from build123d import *

# Parameters (mm, degrees)
SKETCH_1_W           = 20
SKETCH_1_H           = 15
EXTRUDE_1_DEPTH      = 30
EXTRUDE_2_DEPTH      = 6
EXTRUDE_2_DEPTH_BACK = 6
SKETCH_3_R           = 1.35
EXTRUDE_3_DEPTH      = 11.5
EXTRUDE_START        = -0.2
EXTRUDE_4_DEPTH      = 29.6
EXTRUDE_5_DEPTH      = 14.6
FILLET_1_R           = 0.1
FILLET_2_R           = 0.2
SKETCH_6_R           = 1.25
CUT_EXTRUDE_1_DEPTH  = 38.165171868
SKETCH_7_R           = 1.25
CUT_EXTRUDE_2_DEPTH  = 40.449334595
SKETCH_8_R           = 1.25
CUT_EXTRUDE_3_DEPTH  = 5


with BuildPart() as part:
    # 草图1 → 凸台-拉伸1 (new body)
    with BuildSketch(Plane.XY):
        Rectangle(SKETCH_1_W, SKETCH_1_H)
    extrude(amount=-EXTRUDE_1_DEPTH)

    # 草图2 → 凸台-拉伸2 (add, two sides: drawn at the far end of the back side and taken through both)
    with BuildSketch(Plane(origin=(0, 0, 0), x_dir=(1, 0, 0), z_dir=(0, 1, 0)).offset(-EXTRUDE_2_DEPTH_BACK)):
        with BuildLine():
            Line((-4.25, 0), (-5.75, 0))
            Line((-5.75, 0), (-5.75, -0.638562172))
            ThreePointArc((-5.75, -0.638562172), (-5, -2.3), (-4.25, -0.638562172))
            Line((-4.25, -0.638562172), (-4.25, 0))
        make_face()
        with BuildLine():
            Line((4.25, 0), (4.25, -0.638562172))
            ThreePointArc((4.25, -0.638562172), (5, -2.3), (5.75, -0.638562172))
            Line((5.75, -0.638562172), (5.75, 0))
            Line((5.75, 0), (4.25, 0))
        make_face()
    extrude(amount=EXTRUDE_2_DEPTH + EXTRUDE_2_DEPTH_BACK)

    # 草图3 → 凸台-拉伸3 (add)
    with BuildSketch(Plane.XY):
        with Locations(Location((0, 0, 0), (0, 0, 180))):
            Circle(SKETCH_3_R)
    extrude(amount=EXTRUDE_3_DEPTH)

    # 草图4 → 凸台-拉伸4 (add)
    with BuildSketch(Plane.XY.offset(EXTRUDE_START)):
        with BuildLine():
            Line((-1.5, 7.5), (-1.5, 8.177124344))
            ThreePointArc((-1.5, 8.177124344), (-1.780042303, 8.588161527), (-1.95, 9.055590279))
            Line((-1.95, 9.055590279), (-1.95, 10))
            Line((-1.95, 10), (-1.165769145, 10))
            Line((-1.165769145, 10), (-0.5, 8.57225346))
            Line((-0.5, 8.57225346), (-0.5, 7.5))
            Line((-0.5, 7.5), (-1.5, 7.5))
        make_face()
        with BuildLine():
            Line((1.5, 7.5), (1.5, 8.177124344))
            ThreePointArc((1.5, 8.177124344), (1.780042303, 8.588161527), (1.95, 9.055590279))
            Line((1.95, 9.055590279), (1.95, 10))
            Line((1.95, 10), (1.165769145, 10))
            Line((1.165769145, 10), (0.5, 8.57225346))
            Line((0.5, 8.57225346), (0.5, 7.5))
            Line((0.5, 7.5), (1.5, 7.5))
        make_face()
    extrude(amount=-EXTRUDE_4_DEPTH)

    # 草图5 → 凸台-拉伸5 (add)
    with BuildSketch(Plane(origin=(0, 7.5, 0), x_dir=(-1, 0, 0), z_dir=(0, 1, 0)).offset(EXTRUDE_START)):
        with BuildLine():
            Line((1.5, -30), (1.5, -30.677124344))
            ThreePointArc((1.5, -30.677124344), (1.780042303, -31.088161527), (1.95, -31.555590279))
            Line((1.95, -31.555590279), (1.95, -32.5))
            Line((1.95, -32.5), (1.165769145, -32.5))
            Line((1.165769145, -32.5), (0.5, -31.07225346))
            Line((0.5, -31.07225346), (0.5, -30))
            Line((0.5, -30), (1.5, -30))
        make_face()
        with BuildLine():
            Line((-1.5, -30), (-1.5, -30.677124344))
            ThreePointArc((-1.5, -30.677124344), (-1.780042303, -31.088161527), (-1.95, -31.555590279))
            Line((-1.95, -31.555590279), (-1.95, -32.5))
            Line((-1.95, -32.5), (-1.165769145, -32.5))
            Line((-1.165769145, -32.5), (-0.5, -31.07225346))
            Line((-0.5, -31.07225346), (-0.5, -30))
            Line((-0.5, -30), (-1.5, -30))
        make_face()
    extrude(amount=-EXTRUDE_5_DEPTH)

    # 圆角1
    fillet_1_edges = [part.edges().sort_by_distance(p)[0] for p in [
        (-1.557884573, -7.3, -32.5),
        (-1.95, 0, -32.5),
        (-1.165769145, 0, -32.5),
        (-1.557884573, 7.3, -32.5),
        (-1.557884573, 10, -29.8),
        (-1.95, 10, -15),
        (-1.165769145, 10, -15),
        (-1.557884573, 10, -0.2),
        (1.557884573, 10, -29.8),
        (1.165769145, 10, -15),
        (1.95, 10, -15),
        (1.557884573, 10, -0.2),
        (1.557884573, -7.3, -32.5),
        (1.165769145, 0, -32.5),
        (1.95, 0, -32.5),
        (1.557884573, 7.3, -32.5),
    ]]
    fillet(fillet_1_edges, radius=FILLET_1_R)

    # 圆角2
    fillet_2_edges = [part.edges().sort_by_distance(p)[0] for p in [
        (10, 0, -30),
        (0, 7.5, -30),
        (-10, 0, -30),
        (0, 7.5, 0),
        (10, 0, 0),
        (0, -7.5, 0),
        (-10, 0, 0),
        (0, -7.5, -30),
        (-10, 7.5, -15),
        (10, 7.5, -15),
        (10, -7.5, -15),
        (-10, -7.5, -15),
    ]]
    fillet(fillet_2_edges, radius=FILLET_2_R - 0.0001)  # a hair under: the kernel refuses the full size

    # 草图6 → 切除-拉伸1 (cut, through all)
    with BuildSketch(Plane(origin=(0, 7.5, 0), x_dir=(-1, 0, 0), z_dir=(0, 1, 0))):
        with Locations(Location((7.5, -27.5, 0), (0, 0, 90))):
            Circle(SKETCH_6_R)
        with Locations(Location((-7.5, -27.5, 0), (0, 0, 90))):
            Circle(SKETCH_6_R)
    extrude(amount=-CUT_EXTRUDE_1_DEPTH, mode=Mode.SUBTRACT)

    # 草图7 → 切除-拉伸2 (cut, through all)
    with BuildSketch(Plane.ZY.offset(10)):
        with Locations((-27.5, -5)):
            Circle(SKETCH_7_R)
    extrude(amount=-CUT_EXTRUDE_2_DEPTH, mode=Mode.SUBTRACT)

    # 草图8 → 切除-拉伸3 (cut)
    with BuildSketch(Plane(origin=(0, 0, -30), x_dir=(-1, 0, 0), z_dir=(0, 0, -1))):
        with Locations((-7.5, 0)):
            Circle(SKETCH_8_R)
        with Locations((7.5, 0)):
            Circle(SKETCH_8_R)
    extrude(amount=-CUT_EXTRUDE_3_DEPTH, mode=Mode.SUBTRACT)


solid = part.part
Source: CAD feature listing. Evaluate the final solid. Frame: model axes, mm. A direction names the side the tool comes from. Give positions to 0.01 mm unless a question says otherwise; leave off trailing zeros. Order: outer loops, then holes, each group sorted by start corner. A loop starts at its lowest first (then second) coordinate and runs counter-clockwise, first axis right, second up. Notation, with made-up numbers: (6, 69.25) -> (59, 69.25) arc R27 cw to (59, 107.25) -> close; hole circle Ø11 at (30, 40). An arc over 180 degrees is marked (long way). Write item = value, one per line.
Q1. Cut plane D-D, the plane x = -7. Output: boundary loops of the cut face in (y, z).
Data:
outline = (-7.5, -29.8) arc R0.2 ccw to (-7.3, -30) -> (-1.15, -30) -> (-1.15, -28.65) -> (-4.5, -28.65) arc R1.25 cw to (-5.5, -28.65) -> (-7.5, -28.65) -> close; (-7.5, -26.35) -> (-5.5, -26.35) arc R1.25 cw to (-4.5, -26.35) -> (-1.15, -26.35) -> (-1.15, -25) -> (1.15, -25) -> (1.15, -26.35) -> (7.5, -26.35) -> (7.5, -0.2) arc R0.2 ccw to (7.3, 0) -> (-7.3, 0) arc R0.2 ccw to (-7.5, -0.2) -> close; (1.15, -30) -> (7.3, -30) arc R0.2 ccw to (7.5, -29.8) -> (7.5, -28.65) -> (1.15, -28.65) -> close
Q2. Pull-direction query (Y, two-part tool) for faces 4 (the face through (1, -7.3, -31)), 5 (the face through (1.777, 8.582, -14.793)), 6 (the face through (8.421, 0.845, -29.045)), 7 (the face through (-1.777, 0.102, -31.082)); classes: released by +Y, released by -Y, zero draft, split by the parting line, or undercut.
Data:
face_4 = released by -Y
face_5 = undercut
face_6 = undercut
face_7 = zero draft
Q3. Set-up query: faces 1 (the face through (5, -6, 1)), 2 (the face through (-0.824, 9.267, -14.793)), 3 (the face through (8, 0, -25)). Return all of +Z, -Z, +X, -X, +Y, -Y with unobstructed straight access to the full face (end or side cutting, diameter ignored); none if empty.
Data:
face_1 = +Z, +X, -X, -Y
face_2 = +Z, -Z, +Y
face_3 = -Z
Q4. Pin query (flat end, axial travel): pin 1 (2 mm diameter, centred on y = -5, z = -27.5, fed in from +X); pin 2 (0.5 mm diameter, centred on y = 0, z = 0.5, fed in from -X); pin 3 (0.7 mm diameter, centred on x = 1.5, z = -30.5, fed in from -Y); pin 4 (2 mm diameter, centred on x = 7, y = 0, fed in from -Z). Return the tip coordinate at first contact, or that it passes through.
Data:
pin_1 = through
pin_2 = -5.84
pin_3 = -7.3
pin_4 = -30
Q5. Material intervals for line 1 (X direction, y = -1.4, z = -27.5); line 2 (Y direction, x = 7.5, z = -25.5); line 3 (Z direction, x = -7.5, y = 5.75), sorted ascending. Write a range as from..to.
Data:
line_1 = -10..-8.75, -6.25..6.25, 8.75..10
line_2 = -7.5..-1.25, 1.25..7.5
line_3 = -30..-28.75, -26.25..0
Q6. Cut plane C-C, the plane z = -16.5. Output: boundary loops of the cut face in (x, y), and give its area (3 significant figures).
Data:
outline = (-10, -7.3) arc R0.2 ccw to (-9.8, -7.5) -> (9.8, -7.5) arc R0.2 ccw to (10, -7.3) -> (10, 7.3) arc R0.2 ccw to (9.8, 7.5) -> (1.5, 7.5) -> (1.5, 8.18) arc R2 ccw to (1.95, 9.06) -> (1.95, 9.9) arc R0.1 ccw to (1.85, 10) -> (1.23, 10) arc R0.1 ccw to (1.14, 9.94) -> (0.5, 8.57) -> (0.5, 7.5) -> (-0.5, 7.5) -> (-0.5, 8.57) -> (-1.14, 9.94) arc R0.1 ccw to (-1.23, 10) -> (-1.85, 10) arc R0.1 ccw to (-1.95, 9.9) -> (-1.95, 9.06) arc R2 ccw to (-1.5, 8.18) -> (-1.5, 7.5) -> (-9.8, 7.5) arc R0.2 ccw to (-10, 7.3) -> close
area = 305 mm^2
Q7. Cut plane B-B, the plane y = 6.5. Output: boundary loops of the cut face in (x, z).
Data:
outline = (-10, -29.8) arc R0.2 ccw to (-9.8, -30) -> (-1.5, -30) -> (-1.5, -30.68) arc R2 ccw to (-1.95, -31.56) -> (-1.95, -32.4) arc R0.1 ccw to (-1.85, -32.5) -> (-1.23, -32.5) arc R0.1 ccw to (-1.14, -32.44) -> (-0.5, -31.07) -> (-0.5, -30) -> (0.5, -30) -> (0.5, -31.07) -> (1.14, -32.44) arc R0.1 ccw to (1.23, -32.5) -> (1.85, -32.5) arc R0.1 ccw to (1.95, -32.4) -> (1.95, -31.56) arc R2 ccw to (1.5, -30.68) -> (1.5, -30) -> (9.8, -30) arc R0.2 ccw to (10, -29.8) -> (10, -0.2) arc R0.2 ccw to (9.8, 0) -> (-9.8, 0) arc R0.2 ccw to (-10, -0.2) -> close; hole circle Ø2.5 at (-7.5, -27.5); hole circle Ø2.5 at (7.5, -27.5)
Q8. Cut plane A-A, the plane z = 1.3. Output: boundary loops of the cut face in (x, y).
Data:
outline = (-6, -6) -> (-4, -6) -> (-4, 6) -> (-6, 6) -> close; circle Ø2.7 at (0, 0); (4, -6) -> (6, -6) -> (6, 6) -> (4, 6) -> close
